Geometry: see drawing. Coordinates: mm, zero at the bounding-box minimum. A direction names the side the tool comes from. Give positions to 0.01 mm unless a question says otherwise; leave off trailing zeros. Loops run counter-clockwise (first coordinate to the right, second up) from the corner with the lowest first, then second, coordinate; pieces in that order, holes last. Notation, with made-up numbers: (52, 30) -> (100, 30) arc R10 ccw to (100, 37) -> close; hole circle Ø2 at (83, 71). An arc over 180 degrees is marked (long way). Answer in a Markdown table with one row per item. Add a question column.
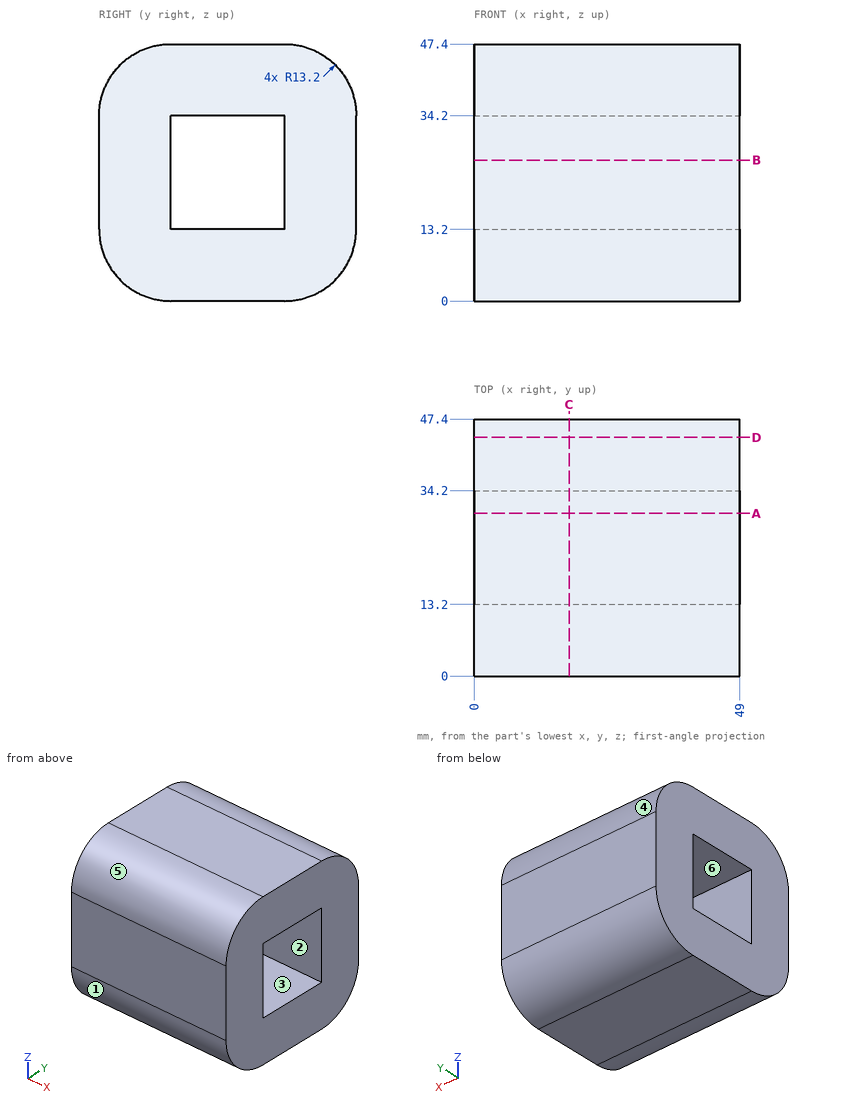
1) Pin query (flat end, axial travel): pin 1 (1 mm diameter, centred on x = 39.5, y = 10.5, fed in from +Z). Return the tip coordinate at first contact, or that it passes through.
2) Section C-C on x = 17.5. Output: boundary loops of the cut face in (y, z).
3) Material intervals for line 1 along Y through (x, z) = (6, 24); line 2 along Z through (x, y) = (30, 13), sorted ascending.
4) Section A-A on y = 30. Output: boundary loops of the cut face in (x, z).
5) Pull-direction query (Y, two-part tool) for the marked faces 3, 4, 5 and 6; classes: +Y half, -Y half, draft (parallel to the pull), parting line (faces both ways), or undercut.
6) Reachability of the marked faces 1 and 2 from +Z, -Z, +X, -X, +Y, -Y: full face, straight path, thin tool, end or side. Return the list, or none.
7) Section D-D on y = 44. Output: boundary loops of the cut face in (x, z).
Working result:
| question | item | result |
|---|---|---|
| 1 | pin 1 | stops at z = 47.22 |
| 2 | outline | (0, 13.2) arc R13.2 ccw to (13.2, 0) -> (34.2, 0) arc R13.2 ccw to (47.4, 13.2) -> (47.4, 34.2) arc R13.2 ccw to (34.2, 47.4) -> (13.2, 47.4) arc R13.2 ccw to (0, 34.2) -> close; hole (13.2, 13.2) -> (34.2, 13.2) -> (34.2, 34.2) -> (13.2, 34.2) -> close |
| 3 | line 1 | y = 0 to 13.2, 34.2 to 47.4 |
| 3 | line 2 | z = 0 to 47.4 |
| 4 | outline | (0, 0) -> (49, 0) -> (49, 13.2) -> (0, 13.2) -> close; (0, 34.2) -> (49, 34.2) -> (49, 47.4) -> (0, 47.4) -> close |
| 5 | face 3 | undercut |
| 5 | face 4 | +Y half |
| 5 | face 5 | -Y half |
| 5 | face 6 | undercut |
| 6 | face 1 | -Z, +X, -X, -Y |
| 6 | face 2 | +X, -X |
| 7 | outline | (0, 4.36) -> (49, 4.36) -> (49, 43.04) -> (0, 43.04) -> close |
